```python
from build123d import *

# Parameters (mm, degrees)
SKETCH_1_W          = 100
SKETCH_1_H          = 60
EXTRUDE_1_DEPTH     = 10
SKETCH_2_R          = 5
CUT_EXTRUDE_1_DEPTH = 20
SKETCH_3_R          = 5
CUT_EXTRUDE_2_DEPTH = 20
CHAMFER_1_SIZE      = 1


with BuildPart() as part:
    # 草图1 → 凸台-拉伸1 (new body)
    with BuildSketch(Plane(origin=(0, 0, 0), x_dir=(1, 0, 0), z_dir=(0, 1, 0))):
        Rectangle(SKETCH_1_W, SKETCH_1_H)
    extrude(amount=EXTRUDE_1_DEPTH)

    # 草图2 → 切除-拉伸1 (cut)
    with BuildSketch(Plane(origin=(0, 0, 0), x_dir=(1, 0, 0), z_dir=(0, 1, 0))):
        with Locations(Location((-20, 0, 0), (0, 0, 90))):
            Circle(SKETCH_2_R)
    extrude(amount=CUT_EXTRUDE_1_DEPTH, mode=Mode.SUBTRACT)

    # 草图3 → 切除-拉伸2 (cut)
    with BuildSketch(Plane(origin=(0, 0, 0), x_dir=(1, 0, 0), z_dir=(0, 1, 0))):
        with Locations(Location((20, 0, 0), (0, 0, 90))):
            Circle(SKETCH_3_R)
    extrude(amount=CUT_EXTRUDE_2_DEPTH, mode=Mode.SUBTRACT)

    # 倒角1
    chamfer_1_edges = [part.edges().sort_by_distance(p)[0] for p in [
        (-20, 0, 5),
        (20, 0, 5),
    ]]
    chamfer(chamfer_1_edges, length=CHAMFER_1_SIZE)


solid = part.part
```
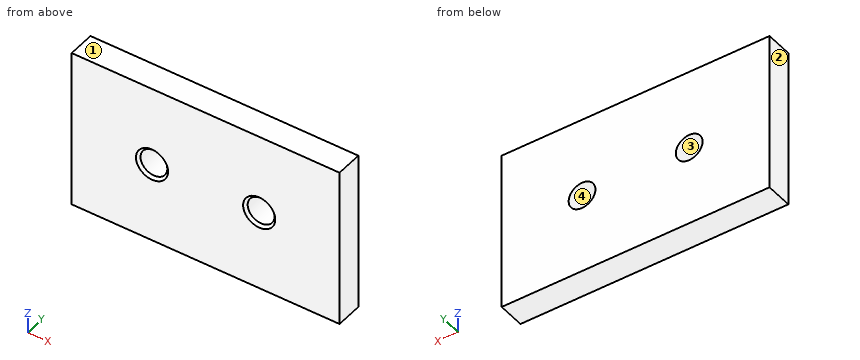
Geometry check sheet. Reference: the model listing, model coordinates, mm. Face numbers are marked on the shaded views. Give positions to 0.01 mm unless a question says otherwise; leave off trailing zeros. Loops run counter-clockwise (first coordinate to the right, second up) from the corner with the lowest first, then second, coordinate; pieces in that order, holes last. Notation, with made-up numbers: (56.5, 35) - (78.5, 35) arc R8 ccw to (78.5, 46) - close; hole circle Ø1 at (-11, -20). An arc over 180 degrees is marked (long way). Use CSV: the item, a comma, the result in double quotes. Start each with the question number.
Q1. Section check B-B, the plane z = 0. Record the cut outline in (x, y).
Q2. Release check for a two-part mould opening along Z. For the marked faces 1, 2, 3 and 4 record: +Z half, -Z half, draft (parallel to the pull), parting line (faces both ways), or undercut.
Q3. Go/stop test with a flat-tipped pin: pin 1 Ø9 at (x, z) = (20, 0) entering from +Y. Record where the tip stops, or that it passes through.
Q4. Scan lines: probe 1 along Z at (x, y) = (-20, 4.25); probe 2 along X at (y, z) = (5, 4); probe 3 along Z at (x, y) = (-21, 3). Record each from-to range of solid material in increasing order. Write a range as from..to.
Q5. Section check A-A, the plane x = -20. Record the cut outline in (y, z), and give its area (3 significant figures).
Q6. Section check C-C, the plane y = 8.5. Record the cut outline in (x, z).
Findings below:
1,outline,"(-50, 0) - (-26, 0) - (-25, 1) - (-25, 10) - (-50, 10) - close; (-15, 1) - (-14, 0) - (14, 0) - (15, 1) - (15, 10) - (-15, 10) - close; (25, 1) - (26, 0) - (50, 0) - (50, 10) - (25, 10) - close"
2,face 1,"+Z half"
2,face 2,"draft"
2,face 3,"undercut"
2,face 4,"undercut"
3,pin 1,"passes through"
4,probe 1,"z = -30..-5, 5..30"
4,probe 2,"x = -50..-23, -17..17, 23..50"
4,probe 3,"z = -30..-4.9, 4.9..30"
5,outline,"(0, -30) - (10, -30) - (10, -5) - (1, -5) - (0, -6) - close; (0, 6) - (1, 5) - (10, 5) - (10, 30) - (0, 30) - close"
5,area,"499 mm^2"
6,outline,"(-50, -30) - (50, -30) - (50, 30) - (-50, 30) - close; hole circle Ø10 at (-20, 0); hole circle Ø10 at (20, 0)"
